The model under review builds one solid part; all positions refer to its coordinate system, in mm. Give positions to 0.01 mm unless a question says otherwise; leave off trailing zeros. Loops run counter-clockwise (first coordinate to the right, second up) from the corner with the lowest first, then second, coordinate; pieces in that order, holes last. Notation, with made-up numbers: (11.25, 50.5) - (37.25, 50.5) arc R15 ccw to (37.25, 73.5) - close; hole circle Ø11 at (1.25, -32.5). An arc over 180 degrees is marked (long way). Answer as a JSON object with one key per item and string values.
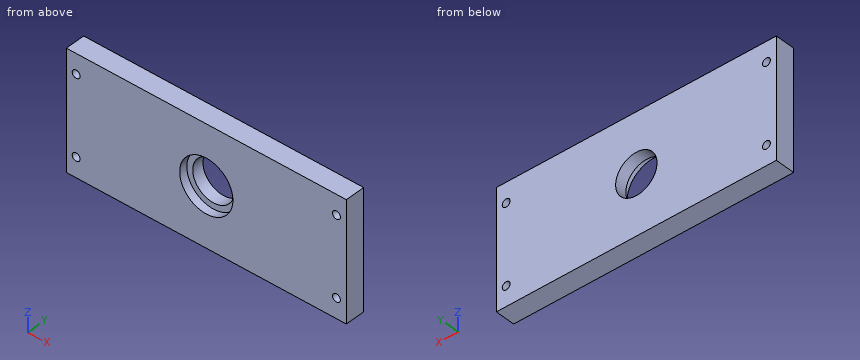
Autodesk Inventor part; units mm, degrees
sketch "スケッチ3" plane through (0, 0, 0) normal (0, 1, 0) x (-1, 0, 0)
  line L0 (71, -30) -> (-71, -30)
  line L1 (-71, -30) -> (-71, 30)
  line L2 (-71, 30) -> (71, 30)
  line L3 (71, 30) -> (71, -30)
  line L4 (71, -30) -> (-71, 30) construction
  line L5 (-71, -30) -> (71, 30) construction
  point P0 (0, 0)
  dimension "d0" = 60
  dimension "d1" = 142
extrude "押し出し1" add sketch "スケッチ3" along normal blind 10
sketch "スケッチ4" plane through (0, 0, 0) normal (0, -1, 0) x (1, 0, 0)
  circle A0 centre (0, 0) radius 13.5
  dimension "d4" = 27
extrude "押し出し2" cut sketch "スケッチ4" against normal blind 4.1
sketch "スケッチ5" plane through (0, 4.1, 0) normal (0, -1, 0) x (1, 0, 0)
  circle A0 centre (0, 0) radius 10.5
  point P0 (0, 0)
  dimension "d7" = 21
extrude "押し出し3" cut sketch "スケッチ5" against normal blind 10
sketch "スケッチ6" plane through (0, 0, 0) normal (0, -1, 0) x (1, 0, 0)
  circle A0 centre (-66, 20) radius 2
  line L0 (-71, 30) -> (-71, -30)
  line L1 (71, 30) -> (-71, 30)
  line L2 (-99.4, 0) -> (99.4, 0)
  circle A1 centre (-66, -20) radius 2
  line L3 (0, -42) -> (0, 42)
  circle A2 centre (66, 20) radius 2
  circle A3 centre (66, -20) radius 2
  point P0 (0, 0)
  dimension "d10" = 4
  dimension "d11" = 5
  dimension "d12" = 10
extrude "押し出し4" cut sketch "スケッチ6" against normal blind 10 contours A0 | A1 | A2 | A3
properties part number "Diffbox_plate_satelite" material "アルミニウム 6061"
Q1. Consider section C-C, the plane x = 0. State the section outline as (y, z) points.
Results:
{"outline": "(0, -30) - (10, -30) - (10, -10.5) - (4.1, -10.5) - (4.1, -13.5) - (0, -13.5) - close; (0, 13.5) - (4.1, 13.5) - (4.1, 10.5) - (10, 10.5) - (10, 30) - (0, 30) - close"}
Q2. Consider section D-D, the plane z = -6. State the section outline as (x, y) points.
Results:
{"outline": "(-71, 0) - (-12.09, 0) - (-12.09, 4.1) - (-8.62, 4.1) - (-8.62, 10) - (-71, 10) - close; (8.62, 4.1) - (12.09, 4.1) - (12.09, 0) - (71, 0) - (71, 10) - (8.62, 10) - close"}
Q3. Consider section A-A, the plane z = -20. State the section outline as (x, y) points, plus the area to 3 significant figures.
Results:
{"outline": "(-71, 0) - (-68, 0) - (-68, 10) - (-71, 10) - close; (-64, 0) - (64, 0) - (64, 10) - (-64, 10) - close; (68, 0) - (71, 0) - (71, 10) - (68, 10) - close", "area": "1,340 mm^2"}
Q4. Consider section B-B, the plane x = -66. State the section outline as (y, z) points.
Results:
{"outline": "(0, -30) - (10, -30) - (10, -22) - (0, -22) - close; (0, -18) - (10, -18) - (10, 18) - (0, 18) - close; (0, 22) - (10, 22) - (10, 30) - (0, 30) - close"}
Q5. Clearance check with flat-ended pins moving along their axes: pin 1 Ø3 at (x, z) = (66, -20) entering from +Y; pin 2 Ø13.5 at (x, z) = (5, 5) entering from -Y; pin 3 Ø5 at (x, z) = (4, 9) entering from -Y. State where each tip first meets the part, or that it passes through.
Results:
{"pin 1": "passes through", "pin 2": "stops at y = 0", "pin 3": "stops at y = 4.1"}
Q6. To check wall thickness, follow probe 1 along Z at (x, y) = (66, 7.75); probe 2 along X at (y, z) = (6.5, -0.5); probe 3 along X at (y, z) = (5.75, 21.5). State the ranges of each line that lie inside material, in increasing order. Write a range as [from, to].
Results:
{"probe 1": "z = [-30, -22], [-18, 18], [22, 30]", "probe 2": "x = [-71, -10.49], [10.49, 71]", "probe 3": "x = [-71, -67.32], [-64.68, 64.68], [67.32, 71]"}
